Source: CAD feature listing. Evaluate the final solid. Frame: model axes, mm. Face numbers are marked on the shaded views. Give positions to 0.01 mm unless a question says otherwise; leave off trailing zeros. Order: outer loops, then holes, each group sorted by start corner. A loop starts at its lowest first (then second) coordinate and runs counter-clockwise, first axis right, second up. Notation, with made-up numbers: (-17, 5) - (5, 5) arc R18 cw to (5, 23) - close; hole circle Ø10 at (18.25, 63.25). An arc over 180 degrees is marked (long way). One line per item, written item: value. Start each with the question number.
from build123d import *

# Parameters (mm, degrees)
SKETCH1_W           = 304.8
SKETCH1_H           = 139.7
BOSS_EXTRUDE1_DEPTH = 12.7
SKETCH5_R           = 1.5
SKETCH5_R_2         = 6.35
CUT_EXTRUDE2_DEPTH  = 13.7
SKETCH8_W           = 44.45
SKETCH8_H           = 44.45
SKETCH8_W_2         = 31.75
SKETCH8_H_2         = 31.75
BOSS_EXTRUDE3_DEPTH = 25.4


with BuildPart() as part:
    # Sketch1 → Boss-Extrude1 (new body)
    with BuildSketch(Plane(origin=(0, 0, 0), x_dir=(1, 0, 0), z_dir=(0, 1, 0))):
        with Locations((152.4, 69.85)):
            Rectangle(SKETCH1_W, SKETCH1_H)
    extrude(amount=BOSS_EXTRUDE1_DEPTH)

    # Sketch5 → Cut-Extrude2 (cut, through all)
    with BuildSketch(Plane(origin=(0, 12.7, 0), x_dir=(1, 0, 0), z_dir=(0, 1, 0))):
        with Locations((165.1, 6.35)):
            Circle(SKETCH5_R)
        with Locations((165.1, 31.75)):
            Circle(SKETCH5_R)
        with Locations((139.7, 31.75)):
            Circle(SKETCH5_R)
        with Locations((12.7, 12.7)):
            Circle(SKETCH5_R_2)
        with Locations((139.7, 6.35)):
            Circle(SKETCH5_R)
        with Locations((292.1, 12.7)):
            Circle(SKETCH5_R_2)
    cut_extrude2 = extrude(amount=-CUT_EXTRUDE2_DEPTH, mode=Mode.SUBTRACT)

    # Sketch8 → Boss-Extrude3 (add)
    with BuildSketch(Plane(origin=(0, 12.7, 0), x_dir=(1, 0, 0), z_dir=(0, 1, 0))):
        with Locations((152.4, 69.85)):
            Rectangle(SKETCH8_W, SKETCH8_H)
        with Locations((152.4, 69.85)):
            Rectangle(SKETCH8_W_2, SKETCH8_H_2, mode=Mode.SUBTRACT)
    extrude(amount=BOSS_EXTRUDE3_DEPTH)

    # Mirror1: Cut-Extrude2 across plane
    add(cut_extrude2.mirror(Plane.XY.offset(-69.85)), mode=Mode.SUBTRACT)


solid = part.part
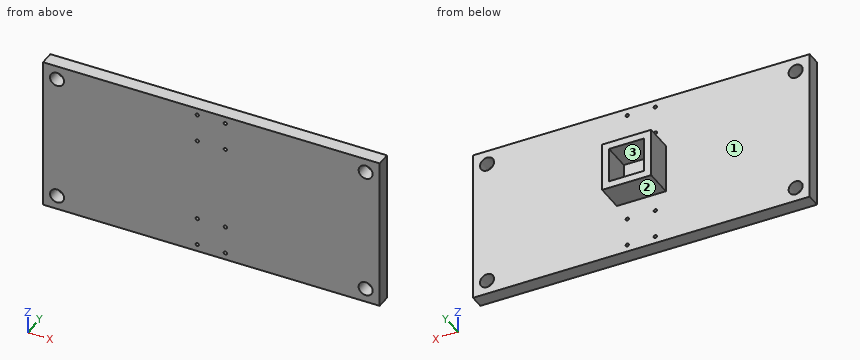
1. Ray query, L1, parallel to X at y = 3, z = -6; L2, parallel to Z at x = 292.1, y = 3.25; L3, parallel to X at y = 14, z = -79.5 (3 decimals). Return the intervals inside material, ascending.
2. Section B-B on y = 24.5. Return the cut outline in (x, z) (3 decimals), then the cut area to 3 significant figures.
3. Section A-A on x = 292.1. Return the cut outline in (y, z).
4. Draft query along Z for the marked faces 1, 2 and 3. Return one class per face: pulls with the +Z half, pulls with the -Z half, needs draft (parallel to the pull), parting line crosses it, or undercut.
5. Section C-C on z = -23. Return the cut outline in (x, y), then the cut area to 3 significant figures.
6. Section D-D on x = 116. Return the cut outline in (y, z).
7. Contact query for flat-ended pins moving along their axis: pin 1 Ø6 at (x, z) = (107, -73) entering from +Y; pin 2 Ø2 at (y, z) = (32.5, -66.5) entering from -X (3 decimals); pin 3 Ø5 at (x, z) = (139.7, -31.75) entering from -Y; pin 4 Ø2.5 at (x, z) = (165.1, -6.35) entering from -Y. Output: stop coordinate, or through.
Data:
1. L1: x = 0 to 138.24, 141.16 to 163.64, 166.56 to 304.8
1. L2: z = -139.7 to -133.35, -120.65 to -19.05, -6.35 to 0
1. L3: x = 130.175 to 136.525, 168.275 to 174.625
2. outline: (130.175, -92.075) - (174.625, -92.075) - (174.625, -47.625) - (130.175, -47.625) - close; hole (136.525, -85.725) - (168.275, -85.725) - (168.275, -53.975) - (136.525, -53.975) - close
2. area: 968 mm2
3. outline: (0, -139.7) - (12.7, -139.7) - (12.7, -133.35) - (0, -133.35) - close; (0, -120.65) - (12.7, -120.65) - (12.7, -19.05) - (0, -19.05) - close; (0, -6.35) - (12.7, -6.35) - (12.7, 0) - (0, 0) - close
4. face 1: needs draft
4. face 2: pulls with the -Z half
4. face 3: undercut
5. outline: (0, 0) - (304.8, 0) - (304.8, 12.7) - (0, 12.7) - close
5. area: 3,870 mm2
6. outline: (0, -139.7) - (12.7, -139.7) - (12.7, 0) - (0, 0) - close
7. pin 1: stops at y = 12.7
7. pin 2: stops at x = 130.175
7. pin 3: stops at y = 0
7. pin 4: passes through
